from build123d import *

# Parameters (mm, degrees)
EXTRUDE_1_DEPTH             = 3.7
EXTRUDE_2_DEPTH             = 1
SKETCH_3_R                  = 17.85
EXTRUDE_3_DEPTH             = 0.5
SKETCH_4_R                  = 18.476621058
EXTRUDE_4_DEPTH             = 7.4
EXTRUDE_5_DEPTH             = 0.85
EXTRUDE_5_DIRECTION_2_REACH = 46.995


with BuildPart() as part:
    # ｽｹｯﾁ1 → ﾎﾞｽ - 押し出し1 (new body)
    with BuildSketch(Plane.XY):
        with BuildLine():
            Line((-12.64, -13.848931367), (-5.089846792, -20.74))
            Line((-5.089846792, -20.74), (5.089846792, -20.74))
            Line((5.089846792, -20.74), (12.64, -13.848931367))
            ThreePointArc((12.64, -13.848931367), (0, 18.75), (-12.64, -13.848931367))
        make_face()
    extrude(amount=-EXTRUDE_1_DEPTH)

    # ｽｹｯﾁ2 → ﾎﾞｽ - 押し出し2 (add)
    with BuildSketch(Plane.XY):
        with BuildLine():
            Line((-14.226252646, -12.968278052), (-8.5, -19.25))
            Line((-8.5, -19.25), (8.5, -19.25))
            Line((8.5, -19.25), (14.226252646, -12.968278052))
            ThreePointArc((14.226252646, -12.968278052), (0, 19.25), (-14.226252646, -12.968278052))
        make_face()
    extrude(amount=EXTRUDE_2_DEPTH)

    # ｽｹｯﾁ3 → ﾎﾞｽ - 押し出し3 (add)
    with BuildSketch(Plane.XY.offset(1)):
        Circle(SKETCH_3_R)
    extrude(amount=EXTRUDE_3_DEPTH)

    # ｽｹｯﾁ4 → ﾎﾞｽ - 押し出し4 (add)
    with BuildSketch(Plane.XY):
        Circle(SKETCH_4_R)
    extrude(amount=-EXTRUDE_4_DEPTH)

    # ｽｹｯﾁ5 → ﾎﾞｽ - 押し出し5 (add)
    with BuildSketch(Plane.XZ.offset(20.74)):
        with BuildLine():
            Line((-2.9, -3.7), (2.9, -3.7))
            ThreePointArc((2.9, -3.7), (4.5, -5.3), (2.9, -6.9))
            Line((2.9, -6.9), (-2.9, -6.9))
            ThreePointArc((-2.9, -6.9), (-4.5, -5.3), (-2.9, -3.7))
        make_face()
    extrude(amount=EXTRUDE_5_DEPTH)

    # ｽｹｯﾁ5 → ﾎﾞｽ - 押し出し5 direction 2 (add, up to next)
    with BuildSketch(Plane.XZ.offset(20.74), mode=Mode.PRIVATE) as extrude_5_direction_2_sk1:
        with BuildLine():
            Line((-2.9, -3.7), (2.9, -3.7))
            ThreePointArc((2.9, -3.7), (4.5, -5.3), (2.9, -6.9))
            Line((2.9, -6.9), (-2.9, -6.9))
            ThreePointArc((-2.9, -6.9), (-4.5, -5.3), (-2.9, -3.7))
        make_face()
    extrude_5_direction_2_tool1 = extrude(extrude_5_direction_2_sk1.sketch, amount=-EXTRUDE_5_DIRECTION_2_REACH, mode=Mode.PRIVATE) - part.part
    add(extrude_5_direction_2_tool1.solids().sort_by_distance((0, -20.74, -5.3))[0])


solid = part.part
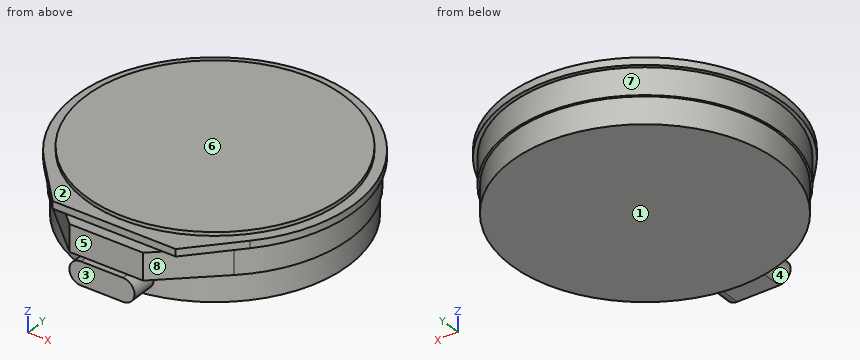
Geometry: final body of the model. Coordinates: model frame, mm. Face numbers are marked on the shaded views. A direction names the side the tool comes from. Give positions to 0.01 mm unless a question says otherwise; leave off trailing zeros. Order: outer loops, then holes, each group sorted by start corner. A loop starts at its lowest first (then second) coordinate and runs counter-clockwise, first axis right, second up. Notation, with made-up numbers: (71.25, 63) -> (95.25, 63) arc R25 cw to (95.25, 96) -> close; hole circle Ø4 at (1, 15.25). An arc over 180 degrees is marked (long way). Answer as a JSON object with one key per item and string values.
Q1. Section C-C (z = -0.75). Output: boundary loops of the cut face in (x, y), plus the area to 3 significant figures.
Entries:
{"outline": "(-12.64, -13.85) -> (-5.09, -20.74) -> (5.09, -20.74) -> (12.64, -13.85) arc R18.75 ccw (long way) to start", "area": "1,140 mm^2"}
Q2. Access query for the marked faces 5, 6, 7 and 8. Directions: +Z, -Z, +X, -X, +Y, -Y. A direction counts if a zero-diameter tool reaches every point of the face in a straight line with its end or side. Return the directions, or none.
Entries:
{"face 5": "+Z, +X, -X, -Y", "face 6": "+Z, +X, -X, +Y, -Y", "face 7": "-Z", "face 8": "-Z, +X, -Y"}
Q3. Section A-A (y = 0). Output: boundary loops of the cut face in (x, z).
Entries:
{"outline": "(-19.25, 0) -> (-18.75, 0) -> (-18.75, -3.7) -> (-18.48, -3.7) -> (-18.48, -7.4) -> (18.48, -7.4) -> (18.48, -3.7) -> (18.75, -3.7) -> (18.75, 0) -> (19.25, 0) -> (19.25, 1) -> (17.85, 1) -> (17.85, 1.5) -> (-17.85, 1.5) -> (-17.85, 1) -> (-19.25, 1) -> close"}
Q4. First-contact query: pin 1 (1.6 mm diameter, centred on x = -3, y = -20, fed in from +Z); pin 2 (1 mm diameter, centred on x = -13.5, z = -5.5, fed in from -Y); pin 3 (5 mm diameter, centred on x = -14, z = -3.5, fed in from +Y). Flat tips, straight axial feed; report the tip coordinate or a pass-through.
Entries:
{"pin 1": "stops at z = 1", "pin 2": "stops at y = -13.13", "pin 3": "stops at y = 14.81"}
Q5. Section D-D (z = -5.3). Output: boundary loops of the cut face in (x, y).
Entries:
{"outline": "(-4.5, -21.59) -> (4.5, -21.59) -> (4.5, -17.92) arc R18.48 ccw (long way) to (-4.5, -17.92) -> close"}
Q6. Draft query along Z for the marked faces 1, 2, 3 and 4. Return one class per face: released by +Z, released by -Z, zero draft, split by the parting line, or undercut.
Entries:
{"face 1": "released by -Z", "face 2": "released by +Z", "face 3": "zero draft", "face 4": "undercut"}
Q7. Material intervals for probe 1 along X at (y, z) = (-0.5, 0.75); probe 2 along Z at (x, y) = (-8, 16); probe 3 along Y at (x, z) = (-4.5, -7), sorted ascending.
Entries:
{"probe 1": "x = -19.24 to 19.24", "probe 2": "z = -7.4 to 1", "probe 3": "y = -17.92 to 17.92"}
